Input: dimensioned drawing with shaded views. Units: mm. Origin: part minimum x, y, z. Coordinates: 2 decimals unless noted, no trailing zeros. Order: outer loops, then holes, each group sorted by start corner. A loop starts at its lowest first (then second) coordinate and runs counter-clockwise, first axis right, second up. Notation, with made-up numbers: (58, 12) - (105, 12) arc R26 cw to (105, 29) - close; hole circle Ø2 at (-23.75, 9). An arc over 180 degrees is marked (long way). Use one line per item in the form item = value. Start each with the question number.
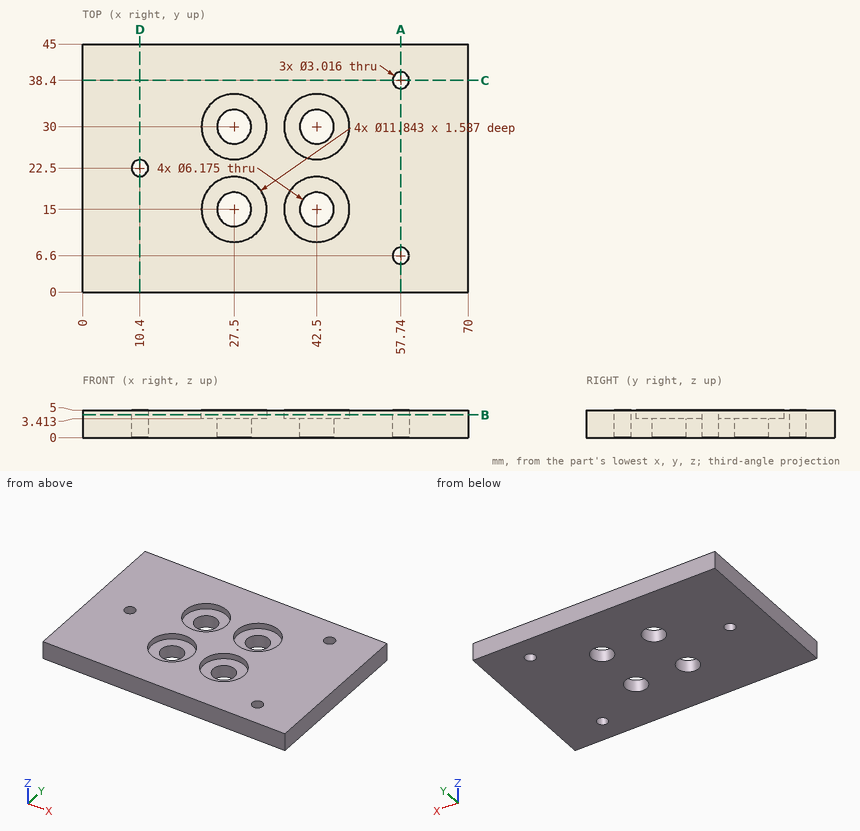
(1) Cut plane B-B on z = 4.15. Return the cut outline in (x, y) (1 decimal).
(2) Material intervals for L1, parallel to Y at x = 57.74, z = 2.8; L2, parallel to Y at x = 42.5, z = 2.6; L3, parallel to X at y = 13.5, z = 0.3, sorted ascending. Write a range as from..to.
(3) Cut plane C-C on y = 38.4. Return the cut outline in (x, z), plus the area to 3 significant figures.
(4) Cut plane A-A on x = 57.74. Return the cut outline in (y, z), plus the area to 3 significant figures.
(5) Cut plane D-D on x = 10.4. Return the cut outline in (y, z).
(6) Contact query for a flat-ended pin moving along its axis: pin 1 Ø3.5 at (x, y) = (29, 15) entering from +Z. Output: stop coordinate, or through.
Check sheet entries:
q1.outline = (0, 0) - (70, 0) - (70, 45) - (0, 45) - close; hole circle Ø3 at (10.4, 22.5); hole circle Ø11.8 at (27.5, 15); hole circle Ø11.8 at (27.5, 30); hole circle Ø11.8 at (42.5, 15); hole circle Ø11.8 at (42.5, 30); hole circle Ø3 at (57.7, 6.6); hole circle Ø3 at (57.7, 38.4)
q2.L1 = 0..5.09, 8.11..36.89, 39.91..45
q2.L2 = 0..11.91, 18.09..26.91, 33.09..45
q2.L3 = 0..24.8, 30.2..39.8, 45.2..70
q3.outline = (0, 0) - (56.23, 0) - (56.23, 5) - (0, 5) - close; (59.25, 0) - (70, 0) - (70, 5) - (59.25, 5) - close
q3.area = 335 mm^2
q4.outline = (0, 0) - (5.09, 0) - (5.09, 5) - (0, 5) - close; (8.11, 0) - (36.89, 0) - (36.89, 5) - (8.11, 5) - close; (39.91, 0) - (45, 0) - (45, 5) - (39.91, 5) - close
q4.area = 195 mm^2
q5.outline = (0, 0) - (20.99, 0) - (20.99, 5) - (0, 5) - close; (24.01, 0) - (45, 0) - (45, 5) - (24.01, 5) - close
q6.pin_1 = 3.41
